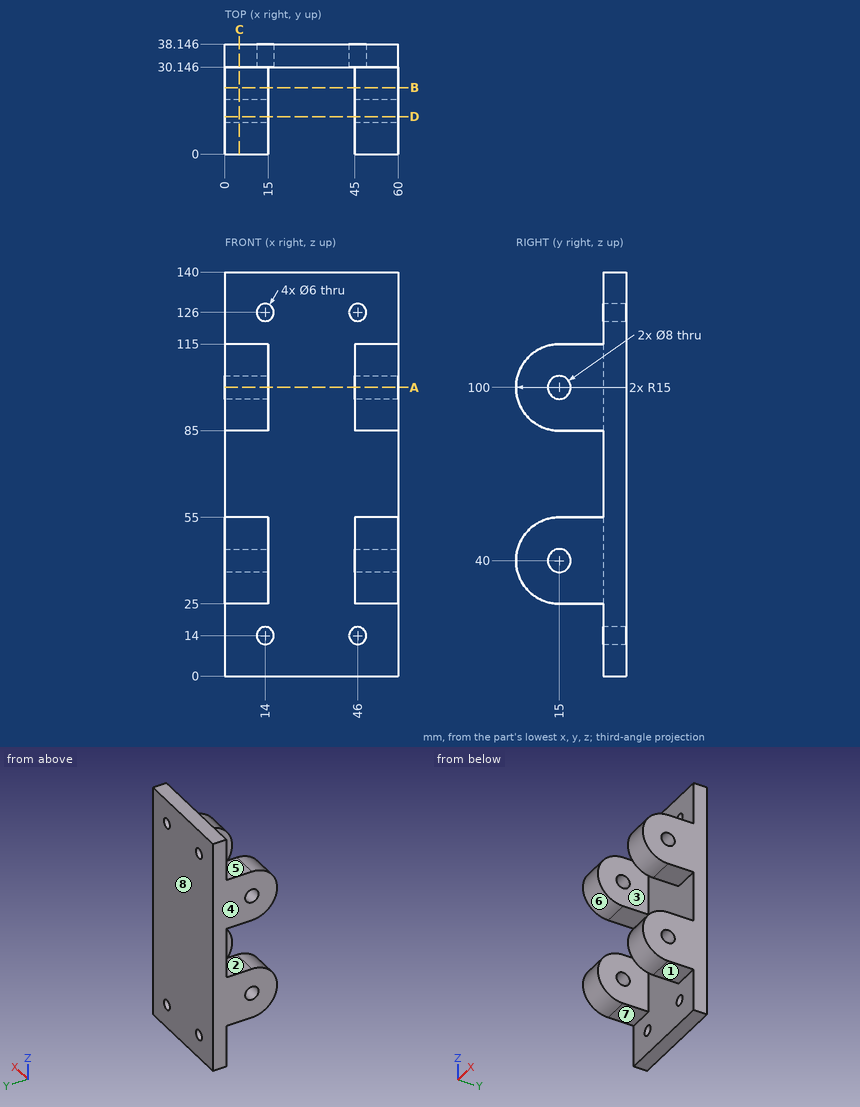
Input: dimensioned drawing with shaded views. Units: mm. Origin: part minimum x, y, z. A direction names the side the tool comes from. Give positions to 0.01 mm unless a question says otherwise; leave off trailing zeros. Write each loop counter-clockwise with the first axis right and the second up, starting at its lowest first coordinate (ties: lowest second). Pieces come first, ordered by that corner, then holes.
1. Section query A-A (z = 100). Return the cut outline in (x, y).
2. Material intervals for line 1 along X through (y, z) = (6, 44); line 2 along X through (y, z) = (33, 126); line 3 along Y through (x, z) = (56.75, 100), sorted ascending.
3. Section query B-B (y = 23). Return the cut outline in (x, z).
4. Pull-direction query (Z, two-part tool) for the marked faces 5, 6, 7 and 8; classes: +Z half, -Z half, draft (parallel to the pull), parting line (faces both ways), or undercut.
5. Access query for the marked faces 1, 2, 3 and 4. Directions: +Z, -Z, +X, -X, +Y, -Y. A direction counts if a zero-diameter tool reaches every point of the face in a straight line with its end or side. Return the directions, or none.
6. Section query D-D (y = 13). Count the separate pieces of the cut face and the enclosed holes in it, then the cut area to 3 significant figures.
7. First-contact query: pin 1 (12 mm diameter, centred on x = 7, y = 21, fed in from -Z); pin 2 (5.5 mm diameter, centred on x = 46, z = 14, fed in from +Y); pin 3 (6 mm diameter, centred on x = 43.5, z = 36.5, fed in from -Y); pin 4 (7.5 mm diameter, centred on x = 53.5, y = 21, fed in from +Z). Flat tips, straight axial feed; report the tip coordinate or a pass-through.
8. Section query C-C (x = 5). Return the cut outline in (y, z), then the cut area to 4 significant figures.
Output values:
1. outline: (0, 0) - (15, 0) - (15, 11) - (0, 11) - close; (0, 19) - (15, 19) - (15, 30.15) - (45, 30.15) - (45, 19) - (60, 19) - (60, 38.15) - (0, 38.15) - close; (45, 0) - (60, 0) - (60, 11) - (45, 11) - close
2. line 1: x = 0 to 15, 45 to 60
2. line 2: x = 0 to 11, 17 to 43, 49 to 60
2. line 3: y = 0 to 11, 19 to 38.15
3. outline: (0, 25) - (15, 25) - (15, 55) - (0, 55) - close; (0, 85) - (15, 85) - (15, 115) - (0, 115) - close; (45, 25) - (60, 25) - (60, 55) - (45, 55) - close; (45, 85) - (60, 85) - (60, 115) - (45, 115) - close
4. face 5: +Z half
4. face 6: undercut
4. face 7: -Z half
4. face 8: draft
5. face 1: -Z, +X, -X, -Y
5. face 2: +X, -X, -Y
5. face 3: +Z, -Z, -Y
5. face 4: +Z, -Z, -X, +Y, -Y
6. separate pieces: 8
6. enclosed holes: 0
6. area: 1,370 mm2
7. pin 1: stops at z = 25
7. pin 2: passes through
7. pin 3: stops at y = 0.03
7. pin 4: stops at z = 115
8. outline: (15, 25) - (30.15, 25) - (30.15, 0) - (38.15, 0) - (38.15, 140) - (30.15, 140) - (30.15, 115) - (15, 115) arc R15 ccw to (15, 85) - (30.15, 85) - (30.15, 55) - (15, 55) arc R15 ccw to start; hole circle Ø8 at (15, 40); hole circle Ø8 at (15, 100)
8. area: 2,635 mm2
